Autodesk Inventor part; units mm, degrees
ref_plane "YZ Plane" through (0, 0, 0) normal (1, 0, 0) x (0, 1, 0)
ref_plane "XZ Plane" through (0, 0, 0) normal (0, 1, 0) x (-1, 0, 0)
ref_plane "XY Plane" through (0, 0, 0) normal (0, 0, 1) x (1, 0, 0)
sketch "Sketch1" plane through (0, 0, 0) normal (0, 0, 1) x (1, 0, 0)
  line L0 (0, 24.5) -> (0, -24.5) construction
  line L1 (-63, 0) -> (63, 0) construction
  line L2 (45, -17.5) -> (-45, -17.5)
  line L3 (-45, -17.5) -> (-45, 17.5)
  line L4 (-45, 17.5) -> (45, 17.5)
  line L5 (45, 17.5) -> (45, -17.5)
  line L6 (45, -17.5) -> (-45, 17.5) construction
  line L7 (-45, -17.5) -> (45, 17.5) construction
  point P0 (0, 0)
  dimension "d0" = 90
  dimension "d1" = 35
extrude "Extrusion1" add sketch "Sketch1" along normal mid plane 0.8
sketch "Esquisse2" plane through (0, 0, 0.4) normal (0, 0, 1) x (1, 0, 0)
  line L0 (-38, 11.5) -> (38, 11.5)
  line L1 (38, 11.5) -> (38, -11.5)
  line L2 (38, -11.5) -> (-38, -11.5)
  line L3 (-38, -11.5) -> (-38, 11.5)
  line L4 (-45, -17.5) -> (45, -17.5) construction
  line L5 (45, -17.5) -> (45, 17.5) construction
  line L6 (45, 17.5) -> (-45, 17.5) construction
  line L7 (-45, 17.5) -> (-45, -17.5) construction
  line L8 (0, 24.5) -> (0, -24.5) construction
  line L9 (-63, 0) -> (63, 0) construction
  point P0 (0, 0)
  dimension "d4" = 76
  dimension "d5" = 23
extrude "Extrusion2" cut sketch "Esquisse2" against normal blind 10
sketch "Esquisse4" plane through (0, 0, -0.4) normal (0, 0, -1) x (-1, 0, 0)
  line L0 (-45, 14.0096) -> (-44.2, 14.0096)
  line L1 (-44.2, 14.0096) -> (-44.2, 6.0096)
  line L2 (-44.2, 6.0096) -> (-45, 6.0096)
  line L3 (-45, 6.0096) -> (-45, 14.0096)
  line L4 (-44.2, -13.9904) -> (-45, -13.9904)
  line L5 (-45, -13.9904) -> (-45, -5.9904)
  line L6 (-45, -5.9904) -> (-44.2, -5.9904)
  line L7 (-44.2, -5.9904) -> (-44.2, -13.9904)
  line L8 (45, -13.9904) -> (44.2, -13.9904)
  line L9 (44.2, -13.9904) -> (44.2, -5.9904)
  line L10 (44.2, -5.9904) -> (45, -5.9904)
  line L11 (45, -5.9904) -> (45, -13.9904)
  line L12 (44.2, 14.0096) -> (45, 14.0096)
  line L13 (45, 14.0096) -> (45, 6.0096)
  line L14 (45, 6.0096) -> (44.2, 6.0096)
  line L15 (44.2, 6.0096) -> (44.2, 14.0096)
  point P0 (0, 0)
extrude "Extrusion4" cut sketch "Esquisse4" against normal blind 0.8
sketch "Esquisse5" plane through (0, 0, 0.4) normal (0, 0, 1) x (1, 0, 0)
  line L0 (-44.2, 14.0096) -> (-45, 14.0096) construction
  line L1 (-45, 14.0096) -> (-45, 17.5) construction
  line L2 (-45, 17.5) -> (45, 17.5) construction
  line L3 (45, 17.5) -> (45, 14.0096) construction
  line L4 (45, 14.0096) -> (44.2, 14.0096) construction
  line L5 (44.2, 14.0096) -> (44.2, 6.0096) construction
  line L6 (44.2, 6.0096) -> (45, 6.0096) construction
  line L7 (45, 6.0096) -> (45, -5.9904) construction
  line L8 (45, -5.9904) -> (44.2, -5.9904) construction
  line L9 (44.2, -5.9904) -> (44.2, -13.9904) construction
  line L10 (44.2, -13.9904) -> (45, -13.9904) construction
  line L11 (45, -13.9904) -> (45, -17.5) construction
  line L12 (45, -17.5) -> (-45, -17.5) construction
  line L13 (-45, -17.5) -> (-45, -13.9904) construction
  line L14 (-45, -13.9904) -> (-44.2, -13.9904) construction
  line L15 (-44.2, -13.9904) -> (-44.2, -5.9904) construction
  line L16 (-44.2, -5.9904) -> (-45, -5.9904) construction
  line L17 (-45, -5.9904) -> (-45, 6.0096) construction
  line L18 (-45, 6.0096) -> (-44.2, 6.0096) construction
  line L19 (-44.2, 6.0096) -> (-44.2, 14.0096) construction
  line L20 (38, -11.5) -> (38, 11.5) construction
  line L21 (38, 11.5) -> (-38, 11.5) construction
  line L22 (-38, 11.5) -> (-38, -11.5) construction
  line L23 (-38, -11.5) -> (38, -11.5) construction
  line L24 (-38, -11.5) -> (-38, 11.5) construction
  line L25 (-38, 11.5) -> (38, 11.5) construction
  line L26 (38, 11.5) -> (38, -11.5) construction
  line L27 (38, -11.5) -> (-38, -11.5) construction
  line L28 (-45, -5.9904) -> (-44.2, -5.9904) construction
  line L29 (-44.2, -5.9904) -> (-44.2, -13.9904) construction
  line L30 (-44.2, -13.9904) -> (-45, -13.9904) construction
  line L31 (-45, -13.9904) -> (-45, -17.5) construction
  line L32 (-45, -17.5) -> (45, -17.5) construction
  line L33 (45, -17.5) -> (45, -13.9904) construction
  line L34 (45, -13.9904) -> (44.2, -13.9904) construction
  line L35 (44.2, -13.9904) -> (44.2, -5.9904) construction
  line L36 (44.2, -5.9904) -> (45, -5.9904) construction
  line L37 (45, -5.9904) -> (45, 6.0096) construction
  line L38 (45, 6.0096) -> (44.2, 6.0096) construction
  line L39 (44.2, 6.0096) -> (44.2, 14.0096) construction
  line L40 (44.2, 14.0096) -> (45, 14.0096) construction
  line L41 (45, 14.0096) -> (45, 17.5) construction
  line L42 (45, 17.5) -> (-45, 17.5) construction
  line L43 (-45, 17.5) -> (-45, 14.0096) construction
  line L44 (-45, 14.0096) -> (-44.2, 14.0096) construction
  line L45 (-44.2, 14.0096) -> (-44.2, 6.0096) construction
  line L46 (-44.2, 6.0096) -> (-45, 6.0096) construction
  line L47 (-45, 6.0096) -> (-45, -5.9904) construction
  line L48 (-63, 0) -> (63, 0) construction
  line L49 (0, 24.66) -> (0, -25.46) construction
  line L50 (-34, -17.5) -> (-26, -17.5)
  line L51 (-26, -17.5) -> (-26, -18.3)
  line L52 (-26, -18.3) -> (-34, -18.3)
  line L53 (-34, -18.3) -> (-34, -17.5)
  line L54 (-4, -18.3) -> (-4, -17.5)
  line L55 (-4, -17.5) -> (4, -17.5)
  line L56 (4, -17.5) -> (4, -18.3)
  line L57 (4, -18.3) -> (-4, -18.3)
  line L58 (26, -18.3) -> (26, -17.5)
  line L59 (26, -17.5) -> (34, -17.5)
  line L60 (34, -17.5) -> (34, -18.3)
  line L61 (34, -18.3) -> (26, -18.3)
  point P0 (0, 0)
  dimension "d32" = 8
  dimension "d33" = 0.8
  dimension "d36" = 30
extrude "Extrusion5" add sketch "Esquisse5" against normal blind 0.8
properties part number "Carosserie_Capot_Avant_Haut" material "PVC-U"
Source: CAD feature listing. Evaluate the final solid. Frame: model axes, mm. Round coordinates to 2 decimals unless told otherwise and drop trailing zeros. Write each loop counter-clockwise with the first axis right and the second up, starting at its lowest first coordinate (ties: lowest second). Pieces come first, ordered by that corner, then holes. Notation, with made-up numbers: (46, -19.5) - (71, -19.5) arc R19 cw to (71, -8.5) - close; hole circle Ø9 at (88, -34.75). An arc over 180 degrees is marked (long way). Use CSV: the item, a comma, the result in double quotes. Start each with the question number.
(1) First-contact query: pin 1 Ø12 at (x, y) = (-28.5, 3) entering from +Z. Flat tip, straight axial feed; report the tip coordinate or a pass-through.
(2) Material intervals for probe 1 along X at (y, z) = (-7, -0.3); probe 2 along Y at (x, z) = (17.5, 0.2); probe 3 along Y at (x, z) = (-30.5, -0.2), sorted ascending. Write a range as [from, to].
(3) Cut plane A-A, the plane x = -24.5. Return loops of the section in (y, z).
(4) Cut plane B-B, the plane y = -4.5. Return loops of the section in (x, z).
(5) Cut plane C-C, the plane y = -13. Return loops of the section in (x, z), and give its area (3 significant figures).
Geometry says:
1,pin 1,"through"
2,probe 1,"[-44.2, -38], [38, 44.2]"
2,probe 2,"[-17.5, -11.5], [11.5, 17.5]"
2,probe 3,"[-18.3, -11.5], [11.5, 17.5]"
3,outline,"(-17.5, -0.4) - (-11.5, -0.4) - (-11.5, 0.4) - (-17.5, 0.4) - close; (11.5, -0.4) - (17.5, -0.4) - (17.5, 0.4) - (11.5, 0.4) - close"
4,outline,"(-45, -0.4) - (-38, -0.4) - (-38, 0.4) - (-45, 0.4) - close; (38, -0.4) - (45, -0.4) - (45, 0.4) - (38, 0.4) - close"
5,outline,"(-44.2, -0.4) - (44.2, -0.4) - (44.2, 0.4) - (-44.2, 0.4) - close"
5,area,"70.7 mm²"
